Solid Edge part; units mm, degrees
sketch "Sketch1" plane through (0, 0, 0) normal (0, -1, 0) x (1, 0, 0)
  line L0 (0, 0) -> (0, 37.5)
  line L1 (0, 37.5) -> (6, 37.5)
  line L2 (6, 37.5) -> (8, 35.5)
  line L3 (8, 35.5) -> (8, 0)
  dimension "D1" = 6
revolve "RevolvedProtrusion1" add sketch "Sketch1" angle 360 about axis through (12, 0, 0) along (-1, 0, 0)
sketch "Sketch2" plane through (8, 0, 0) normal (1, 0, 0) x (0, 1, 0)
  line L0 (-30, 4) -> (-30, -4)
  line L1 (-30, -4) -> (30, -4)
  line L2 (30, -4) -> (30, 4)
  line L3 (30, 4) -> (-30, 4)
  line L4 (-30, -12) -> (30, -12)
  line L5 (30, -12) -> (30, -18)
  line L6 (30, -18) -> (-30, -18)
  line L7 (-30, -18) -> (-30, -12)
  dimension "D1" = 30
  dimension "D2" = 30
  dimension "D3" = 30
extrude "Protrusion1" add sketch "Sketch2" along normal blind 30
sketch "Sketch3" plane through (25, 0, 4) normal (0, 0, 1) x (0, 1, 0)
  line L0 (-20.5, -8.5) -> (20.5, -8.5)
  line L1 (20.5, -8.5) -> (20.5, 12.5)
  line L2 (20.5, 12.5) -> (-20.5, 12.5)
  line L3 (-20.5, 12.5) -> (-20.5, -8.5)
  dimension "D1" = 20.5
  dimension "D2" = 20.5
extrude "ExtrudedCutout_1" cut sketch "Sketch3" against normal blind 6
hole "Hole_1" at (23, -10, -18) direction (0, 0, 1) diameter 4 end up to next
hole "Hole1" at (23, 10, -18) direction (0, 0, 1) diameter 4 end up to next
sketch "Sketch4" plane through (23, 0, 4) normal (1, 0, 0) x (0, 1, 0)
  line L0 (10, -6) -> (17.5, -6)
  line L1 (17.5, -6) -> (17.5, -8.5)
  line L2 (17.5, -8.5) -> (14, -8.5)
  line L3 (14, -8.5) -> (14, -8)
  line L4 (14, -8) -> (10, -8)
  dimension "D1" = 17.5
  dimension "D2" = 10
revolve "RevolvedCutout1" cut sketch "Sketch4" angle 360 about axis through (23, 10, -2) along (0, 0, 1)
hole "Hole_3" at (18, -25, 4) direction (0, 0, -1) diameter 3 end up to next
hole "Hole2" at (28, -25, 4) direction (0, 0, -1) diameter 3 end up to next
hole "Hole_5" at (8, 0, -30) direction (-1, 0, 0) diameter 4.8 end up to next counterbore diameter 8 counterbore depth 4.8
hole "Hole3" at (8, -30, 10) direction (-1, 0, 0) diameter 4.8 end up to next counterbore diameter 8 counterbore depth 4.8
hole "Hole4" at (8, 30, 10) direction (-1, 0, 0) diameter 4.8 end up to next counterbore diameter 8 counterbore depth 4.8
sketch "Sketch5" plane through (8, 0, 20.75) normal (1, 0, 0) x (0, 1, 0)
  line L0 (-38.8569, 19.7387) -> (38.8569, 19.7387)
  line L1 (38.8569, 19.7387) -> (38.8569, -3.25)
  line L2 (38.8569, -3.25) -> (-38.8569, -3.25)
  line L3 (-38.8569, -3.25) -> (-38.8569, 19.7387)
extrude "ExtrudedCutout_2" cut sketch "Sketch5" against normal blind 180
chamfer "Chamfer_1" distance 2 angle 45 1 edges at (8, 0, 17.5)
chamfer "Chamfer_2" distance 1 angle 45 10 edges at (23, -30, -18) (38, 0, -18) (23, 30, -18) (38, 30, -15) (38, 30, 0) (23, 30, 4) (38, 0, 4) (23, -30, 4) (38, -30, 0) (38, -30, -15)
hole "Hole_10" at (23, -10, -4) direction (0, 0, 1) diameter 4 end up to next
mirror "Mirror1" about plane through (0, 0, 0) normal (0, -1, 0) of "Hole_3", "Hole2"
properties material "Polyethylene, low density"
Check sheet for the modelled part. Datum: model origin and axes. Units: mm. A direction names the side the tool comes from. Round coordinates to 2 decimals unless told otherwise and drop trailing zeros. Order: outer loops, then holes, each group sorted by start corner. A loop starts at its lowest first (then second) coordinate and runs counter-clockwise, first axis right, second up.
Q1. Cross-section at A-A, the plane y = 0. Enter the section's corners in (x, z), plus the area to 3 significant figures.
Filled sheet:
outline: (0, -37.5) - (6, -37.5) - (8, -35.5) - (8, -34) - (3.2, -34) - (3.2, -32.4) - (0, -32.4) - close; (0, -27.6) - (3.2, -27.6) - (3.2, -26) - (8, -26) - (8, -18) - (37, -18) - (38, -17) - (38, -12) - (8, -12) - (8, -4) - (38, -4) - (38, 3) - (37, 4) - (33.5, 4) - (33.5, -2) - (12.5, -2) - (12.5, 4) - (8, 4) - (8, 15.5) - (6, 17.5) - (0, 17.5) - close
area: 675 mm2
Q2. Set-up check for faces 1 (the face through (22, -30, -15)), 2 (the face through (22, 30, -14)), 3 (the face through (3.2, -28, 8)): record each of +Z, -Z, +X, -X, +Y, -Y from which the full face is reachable in a straight line by a thin tool's end or side.
Filled sheet:
face 1: +Z, -Z, +X, -Y
face 2: +Z, -Z, +X, +Y
face 3: +X
Q3. Cross-section at C-C, the plane x = 28. Enter the section's corners in (y, z), plus the area to 3 significant figures.
Filled sheet:
outline: (-30, -17) - (-29, -18) - (29, -18) - (30, -17) - (30, -12) - (-30, -12) - close; (-30, -4) - (-26.5, -4) - (-26.5, 4) - (-29, 4) - (-30, 3) - close; (-23.5, -4) - (4.41, -4) - (4.41, -2) - (-20.5, -2) - (-20.5, 4) - (-23.5, 4) - close; (15.59, -4) - (23.5, -4) - (23.5, 4) - (20.5, 4) - (20.5, -2) - (15.59, -2) - close; (26.5, -4) - (30, -4) - (30, 3) - (29, 4) - (26.5, 4) - close
area: 522 mm2
Q4. Scan lines: L1, parallel to Y at x = 28, z = 1.75; L2, parallel to X at y = 25, z = 0.75; L3, parallel to Z at x = 26, y = 27. Record each from-to range of solid material in increasing order.
Filled sheet:
L1: y = -30 to -26.5, -23.5 to -20.5, 20.5 to 23.5, 26.5 to 30
L2: x = 0 to 16.5, 19.5 to 26.5, 29.5 to 38
L3: z = -18 to -12, -4 to 4
Q5. Draft check along Y on faces 4 (the face through (3.2, 32, 8)), 5 (the face through (23, 0, -4)), 6 (the face through (7.875, 1.025, -35.61)). Enter one of: pulls with the +Y half, pulls with the -Y half, needs draft (parallel to the pull), parting line crosses it, or undercut.
Filled sheet:
face 4: undercut
face 5: needs draft
face 6: parting line crosses it
Q6. Depth check by flat-ended pin: P1, Ø6, axis at y = -24, z = -26.5, coming from the +X side; P2, Ø5, axis at x = 23, y = 10, coming from the -Z side; P3, Ø2, axis at x = 33.5, z = -13.5, coming from the +Y side. Enter the tip coordinate at first touch or a pass-through.
Filled sheet:
P1: stops at x = 8
P2: stops at z = -18
P3: stops at y = 30
Q7. Cross-section at D-D, the plane x = 5. Enter the section's corners in (y, z).
Filled sheet:
outline: (-33.17, 17.5) arc R37.5 ccw (long way) to (33.17, 17.5) - close; hole circle Ø8 at (-30, 10); hole circle Ø8 at (0, -30); hole circle Ø8 at (30, 10)
Q8. Cross-section at B-B, the plane z = 0. Enter the section's corners in (x, y), plus the area to 3 significant figures.
Filled sheet:
outline: (0, -37.5) - (6, -37.5) - (8, -35.5) - (8, -30) - (37, -30) - (38, -29) - (38, 29) - (37, 30) - (8, 30) - (8, 35.5) - (6, 37.5) - (0, 37.5) - close; hole (12.5, -20.5) - (33.5, -20.5) - (33.5, 20.5) - (12.5, 20.5) - close; hole circle Ø3 at (18, -25); hole circle Ø3 at (18, 25); hole circle Ø3 at (28, -25); hole circle Ø3 at (28, 25)
area: 1,510 mm2
